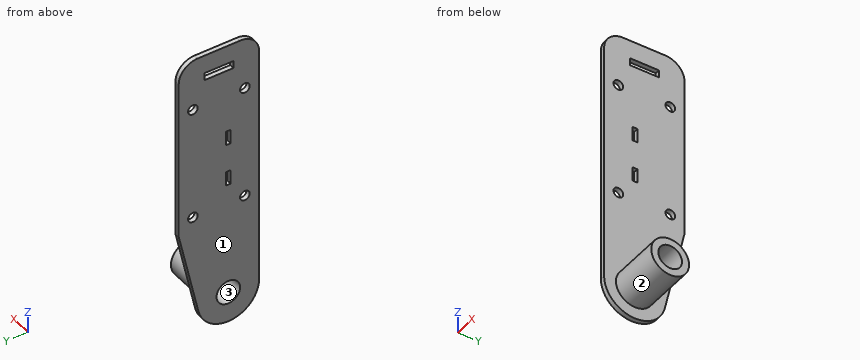
```python
from build123d import *

# Parameters (mm, degrees)
SKETCH1_R           = 3.2639
SKETCH1_R_2         = 12.7
BOSS_EXTRUDE1_DEPTH = 3.175
SKETCH2_R           = 12.7
SKETCH2_R_2         = 7.9375
BOSS_EXTRUDE2_DEPTH = 38.1
SKETCH4_W           = 4.953
SKETCH4_H           = 19.558
BOSS_EXTRUDE3_DEPTH = 3.175
SKETCH5_W           = 9.525
SKETCH5_H           = 3.302
CUT_EXTRUDE1_DEPTH  = 4.175


with BuildPart() as part:
    # Sketch1 → Boss-Extrude1 (new body)
    with BuildSketch(Plane(origin=(0, 0, 0), x_dir=(0, 0, -1), z_dir=(1, 0, 0))):
        with BuildLine():
            Line((106.143178695, 13.781217887), (47.625, 26.9875))
            Line((47.625, 26.9875), (-47.625, 26.9875))
            Line((-47.625, 26.9875), (-47.625, -26.9875))
            Line((-47.625, -26.9875), (101.6, -26.9875))
            ThreePointArc((101.6, -26.9875), (122.110538942, -8.635650576), (106.143178695, 13.781217887))
        make_face()
        with Locations((38.1, 17.4625)):
            Circle(SKETCH1_R, mode=Mode.SUBTRACT)
        with Locations((38.1, -17.4625)):
            Circle(SKETCH1_R, mode=Mode.SUBTRACT)
        with Locations((-38.1, -17.4625)):
            Circle(SKETCH1_R, mode=Mode.SUBTRACT)
        with Locations((-38.1, 17.4625)):
            Circle(SKETCH1_R, mode=Mode.SUBTRACT)
        with Locations((101.6, -6.35)):
            Circle(SKETCH1_R_2, mode=Mode.SUBTRACT)
    extrude(amount=BOSS_EXTRUDE1_DEPTH)

    # Sketch2 → Boss-Extrude2 (add)
    with BuildSketch(Plane.ZY):
        with Locations((-101.6, -6.35)):
            Circle(SKETCH2_R)
        with Locations((-101.6, -6.35)):
            Circle(SKETCH2_R_2, mode=Mode.SUBTRACT)
    extrude(amount=-BOSS_EXTRUDE2_DEPTH)

    # Sketch4 → Boss-Extrude3 (add)
    with BuildSketch(Plane(origin=(3.175, 0, 0), x_dir=(0, 0, -1), z_dir=(1, 0, 0))):
        with BuildLine():
            Line((-47.625, 26.9875), (-60.325, 26.9875))
            ThreePointArc((-60.325, 26.9875), (-69.305256121, 23.267756121), (-73.025, 14.2875))
            Line((-73.025, 14.2875), (-73.025, -14.2875))
            ThreePointArc((-73.025, -14.2875), (-69.305256121, -23.267756121), (-60.325, -26.9875))
            Line((-60.325, -26.9875), (-47.625, -26.9875))
            Line((-47.625, -26.9875), (-47.625, 26.9875))
        make_face()
        with Locations((-58.1025, 0)):
            Rectangle(SKETCH4_W, SKETCH4_H, mode=Mode.SUBTRACT)
    extrude(amount=-BOSS_EXTRUDE3_DEPTH)

    # Sketch5 → Cut-Extrude1 (cut, through all)
    with BuildSketch(Plane(origin=(3.175, 0, 0), x_dir=(0, 0, -1), z_dir=(1, 0, 0))):
        with Locations((20.6375, -6.2865)):
            Rectangle(SKETCH5_W, SKETCH5_H)
        with Locations((-7.9375, -6.2865)):
            Rectangle(SKETCH5_W, SKETCH5_H)
    extrude(amount=-CUT_EXTRUDE1_DEPTH, mode=Mode.SUBTRACT)


solid = part.part
```
The listing builds one solid part. Answer for the finished solid, in the listing's coordinates (mm). Face numbers are marked on the shaded views. Round coordinates to 2 decimals unless told otherwise and drop trailing zeros. Loops run counter-clockwise (first coordinate to the right, second up) from the corner with the lowest first, then second, coordinate; pieces in that order, holes last. Notation, with made-up numbers: (-15.75, -34.5) - (25.25, -34.5) arc R23 ccw to (25.25, -20.5) - close; hole circle Ø2 at (88, 69). An arc over 180 degrees is marked (long way). Use one line per item in the form item = value. Start each with the question number.
1. The part is cut by section D-D on z = 39.5. Determine the outline of the cut face in (x, y) (1 decimal), then the cut area to 3 significant figures.
2. The part is cut by section A-A on z = 8. Determine the outline of the cut face in (x, y) (1 decimal), then the cut area to 3 significant figures.
3. Consider line 1 (Y direction, x = 0.75, z = -38.1); line 2 (Y direction, x = 15, z = -101); line 3 (X direction, y = 18, z = -84) (3 decimals). Determine where each line is inside the solid, lowest interval first. Write a range as [from, to].
4. The part is cut by section B-B on z = -38.1. Determine the outline of the cut face in (x, y) (1 decimal), then the cut area to 3 significant figures.
5. For a pull along Y with two mould halves and no side action, classify the marked faces 1, 2 and 3 as pulls with the +Y half, pulls with the -Y half, needs draft (parallel to the pull), parting line crosses it, or undercut.
6. Given pin 1 Ø1.6 at (x, y) = (2, 1) entering from -Z; pin 2 Ø10 at (x, z) = (10, -27.5) entering from +Y; pin 3 Ø8 at (y, z) = (2.5, 29) entering from +X (3 decimals); pin 4 Ø1.5 at (x, y) = (13, 1) entering from +Z, each flat-ended and moving along its own axis, determine where each tip first touches the part or whether it passes through.
Geometry check:
q1.outline = (0, -27) - (3.2, -27) - (3.2, -20.4) - (0, -20.4) - close; (0, -14.5) - (3.2, -14.5) - (3.2, 14.5) - (0, 14.5) - close; (0, 20.4) - (3.2, 20.4) - (3.2, 27) - (0, 27) - close
q1.area = 134 mm^2
q2.outline = (0, -27) - (3.2, -27) - (3.2, -7.9) - (0, -7.9) - close; (0, -4.6) - (3.2, -4.6) - (3.2, 27) - (0, 27) - close
q2.area = 161 mm^2
q3.line_1 = [-26.99, -20.73], [-14.2, 14.2], [20.73, 26.99]
q3.line_2 = [-19.04, -14.26], [1.56, 6.34]
q3.line_3 = [0, 3.175]
q4.outline = (0, -27) - (3.2, -27) - (3.2, -20.7) - (0, -20.7) - close; (0, -14.2) - (3.2, -14.2) - (3.2, 14.2) - (0, 14.2) - close; (0, 20.7) - (3.2, 20.7) - (3.2, 27) - (0, 27) - close
q4.area = 130 mm^2
q5.face_1 = needs draft
q5.face_2 = parting line crosses it
q5.face_3 = undercut
q6.pin_1 = -121.17
q6.pin_2 = through
q6.pin_3 = 3.175
q6.pin_4 = -90.75
